Geometry: see drawing. Coordinates: mm, zero at the bounding-box minimum. A direction names the side the tool comes from. Round coordinates to 2 decimals unless told otherwise and drop trailing zeros. Loops run counter-clockwise (first coordinate to the right, second up) from the corner with the lowest first, then second, coordinate; pieces in that order, holes last. Notation, with made-up numbers: (69.25, 4) -> (114.25, 4) arc R20 ccw to (114.25, 29) -> close; hole circle Ø11 at (-28.75, 52.5). An arc over 180 degrees is marked (long way). Answer in a Markdown table with one row per item.
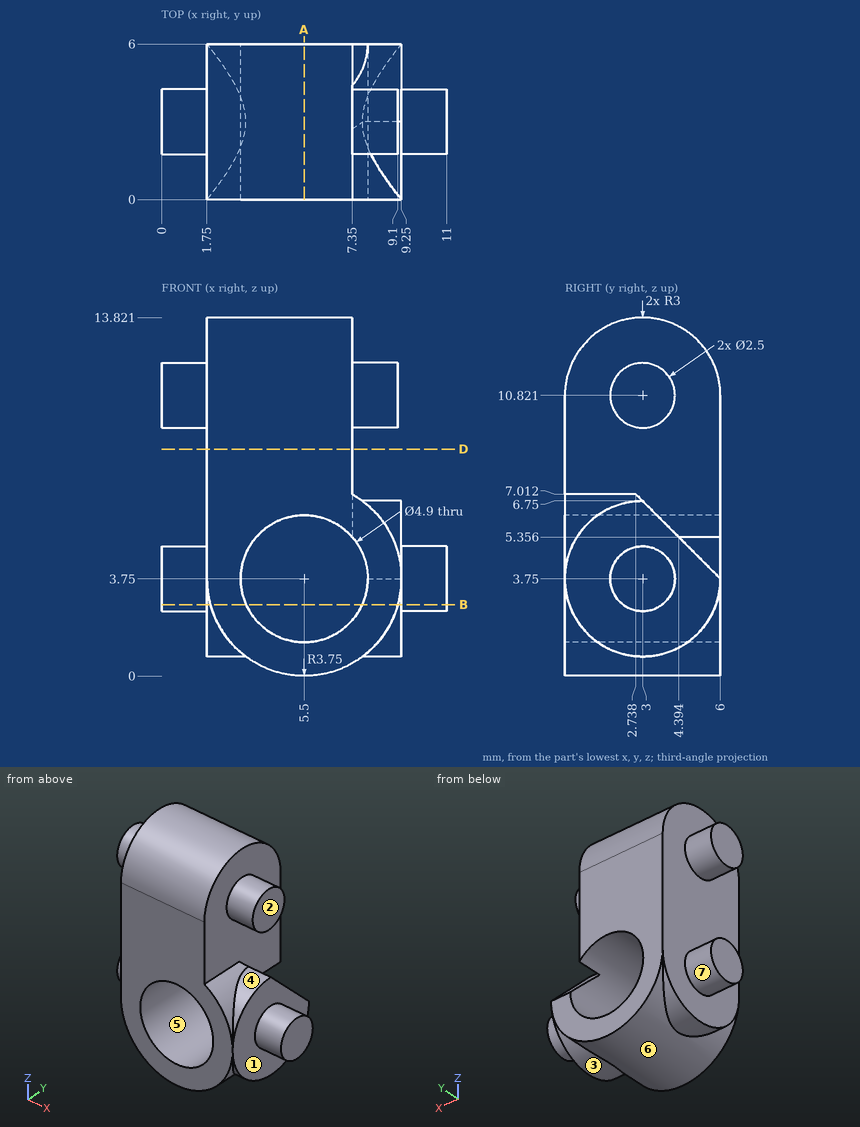
Item 1: Mould query, pull axis X, two halves, no side actions, for the marked faces 5, 6 and 7. Classes: released by +X, released by -X, zero draft, split by the parting line, or undercut.
Ans:
| item | result |
|---|---|
| face 5 | undercut |
| face 6 | split by the parting line |
| face 7 | zero draft |
Item 2: First-contact query: P1, Ø1, axis at x = 10, y = 5.5, coming from the -Z side; P2, Ø3, axis at y = 3.5, z = 10, coming from the +X side; P3, Ø2, axis at y = 2, z = 3, coming from the -X side. Flat tips, straight axial feed; report the tip coordinate or a pass-through.
Ans:
| item | result |
|---|---|
| P1 | through |
| P2 | x = 9.1 |
| P3 | x = 0 |
Item 3: Section query D-D, the plane z = 8.75. Output: boundary loops of the cut face in (x, y).
Ans:
| item | result |
|---|---|
| outline | (1.75, 0) -> (7.35, 0) -> (7.35, 6) -> (1.75, 6) -> close |
Item 4: Section query A-A, the plane x = 5.5. Output: boundary loops of the cut face in (y, z).
Ans:
| item | result |
|---|---|
| outline | (0, 0) -> (6, 0) -> (6, 1.3) -> (0, 1.3) -> close; (0, 6.2) -> (6, 6.2) -> (6, 10.82) arc R3 ccw to (0, 10.82) -> close |
Item 5: Set-up query: the marked faces 1, 2, 3 and 4. Return all of +Z, -Z, +X, -X, +Y, -Y with unobstructed straight access to the full face (end or side cutting, diameter ignored); none if empty.
Ans:
| item | result |
|---|---|
| face 1 | +X |
| face 2 | +Z, +X, +Y, -Y |
| face 3 | -Z, +X |
| face 4 | +X, -Y |
Item 6: Section query B-B, the plane z = 2.75. Output: boundary loops of the cut face in (x, y), and give its area (3 significant figures).
Ans:
| item | result |
|---|---|
| outline | (0, 2.25) -> (1.75, 2.25) -> (1.75, 0.17) -> (1.89, 0.17) -> (1.89, 0) -> (3.26, 0) -> (3.26, 6) -> (1.89, 6) -> (1.89, 5.83) -> (1.75, 5.83) -> (1.75, 3.75) -> (0, 3.75) -> close; (7.74, 0) -> (9.11, 0) -> (9.11, 0.17) -> (9.25, 0.17) -> (9.25, 2.25) -> (11, 2.25) -> (11, 3.75) -> (9.25, 3.75) -> (9.25, 5.83) -> (9.11, 5.83) -> (9.11, 6) -> (7.74, 6) -> close |
| area | 23.3 mm2 |
Item 7: Ray query, L1, parallel to Z at x = 5.5, y = 3.2; L2, parallel to Z at x = 3.75, y = 5.25 (1 decimal); L3, parallel to X at y = 1.5, z = 0.75. Return the intervals inside material, ascending.
Ans:
| item | result |
|---|---|
| L1 | 0 to 1.3, 6.2 to 13.81 |
| L2 | 0.4 to 2, 5.5 to 12.8 |
| L3 | 3.25 to 7.75 |
